Model file for the job. Use its own axes, mm. A direction names the side the tool comes from. Coordinates: 2 decimals unless noted, no trailing zeros. Order: outer loops, then holes, each group sorted by start corner. A loop starts at its lowest first (then second) coordinate and runs counter-clockwise, first axis right, second up. Notation, with made-up numbers: M 2.25,68 L 13.25,68 A12 cw 13.25,81 Z; hole C -8,51 d4. An arc over 180 degrees is marked long. Return JSON: item names as keys, results as strings.
Autodesk Inventor part; units mm, degrees
ref_plane "YZ Plane" through (0, 0, 0) normal (1, 0, 0) x (0, 1, 0)
ref_plane "XZ Plane" through (0, 0, 0) normal (0, 1, 0) x (-1, 0, 0)
ref_plane "XY Plane" through (0, 0, 0) normal (0, 0, 1) x (1, 0, 0)
sketch "Sketch1" plane through (0, 0, 0) normal (0, 1, 0) x (-1, 0, 0)
  circle A0 centre (0, 0) radius 11.5
  circle A1 centre (0, -22) radius 4.25
  line L0 (-21.5, 21.5) -> (21.5, 21.5)
  line L1 (21.5, 21.5) -> (21.5, -21.5)
  line L2 (21.5, -21.5) -> (-21.5, -21.5)
  line L3 (-21.5, -21.5) -> (-21.5, 21.5)
  line L4 (-21.5, 21.5) -> (21.5, -21.5) construction
  line L5 (21.5, 21.5) -> (-21.5, -21.5) construction
  line L6 (21.5, -21.5) -> (-21.5, -21.5)
  line L7 (-21.5, -21.5) -> (-21.5, -29.5)
  line L8 (-21.5, -29.5) -> (21.5, -29.5)
  line L9 (21.5, -29.5) -> (21.5, -21.5)
  circle A2 centre (15.5, 15.5) radius 1.8
  circle A3 centre (15.5, -15.5) radius 1.8
  circle A4 centre (-15.5, -15.5) radius 1.8
  circle A5 centre (-15.5, 15.5) radius 1.8
  point P0 (0, 0)
  dimension "d0" = 23
  dimension "d1" = 22
  dimension "d2" = 8.5
  dimension "d3" = 43
  dimension "d4" = 43
  dimension "d5" = 3.6
  dimension "d6" = 31
  dimension "d7" = 31
  dimension "d8" = 8
extrude "Extrusion1" add sketch "Sketch1" along normal blind 6 contours A1 L2 L9 L8 L7 | A1 L2 L3 L0 L1
sketch "Sketch2" plane through (0, 6, 0) normal (0, 1, 0) x (1, 0, 0)
  line L0 (-21.5, 29.5) -> (-21.5, -21.5)
  line L1 (-21.5, -21.5) -> (-26.5, -21.5)
  line L2 (-26.5, -21.5) -> (-26.5, 29.5)
  line L3 (-26.5, 29.5) -> (-21.5, 29.5)
  line L4 (-21.5, 29.5) -> (-21.5, -21.5)
  line L5 (21.5, -21.5) -> (26.5, -21.5)
  line L6 (26.5, -21.5) -> (26.5, 29.5)
  line L7 (26.5, 29.5) -> (21.5, 29.5)
  line L8 (21.5, 29.5) -> (21.5, -21.5)
  line L9 (-26.5, 29.5) -> (26.5, 29.5)
  line L10 (26.5, 29.5) -> (26.5, 24.5)
  line L11 (26.5, 24.5) -> (-26.5, 24.5)
  line L12 (-26.5, 24.5) -> (-26.5, 29.5)
  circle A0 centre (0, 22) radius 4.25
  line L13 (21.5, 29.5) -> (-21.5, 29.5)
  point P0 (0, 0)
  point P1 (-21.5, 24.5)
  point P2 (-3.4369, 24.5)
  point P3 (3.4369, 24.5)
  point P4 (21.5, 24.5)
  point P5 (21.5, 29.5)
  dimension "d11" = 5
  dimension "d12" = 5
  dimension "d13" = 5
extrude "Extrusion2" add sketch "Sketch2" against normal blind 43.081 contours L9 L8 L11 A0 L0 | L0 L11 L2 L3 | L0 L1 L2 L11 | L7 L6 L11 L8 | L11 L6 L5 L8
sketch "Sketch4" plane through (0, -37.081, 0) normal (0, -1, 0) x (1, 0, 0)
  line L0 (-26.5, 21.5) -> (26.5, 21.5)
  line L1 (26.5, 21.5) -> (41.5, 21.5)
  line L2 (41.5, 21.5) -> (41.5, -29.5)
  line L3 (41.5, -29.5) -> (26.5, -29.5)
  line L4 (26.5, -29.5) -> (26.5, 21.5)
  line L5 (-26.5, -29.5) -> (-26.5, 21.5)
  line L6 (-26.5, 21.5) -> (-41.5, 21.5)
  line L7 (-41.5, 21.5) -> (-41.5, -29.5)
  line L8 (-41.5, -29.5) -> (-26.5, -29.5)
  line L9 (-26.5, -29.5) -> (-26.5, 21.5)
  line L10 (-26.5, -29.5) -> (26.5, -29.5)
  circle A0 centre (-34, -5.25) radius 2.75
  circle A1 centre (34, -5.25) radius 2.75
  point P0 (0, 0)
  point P1 (-26.5, -29.5)
  dimension "d21" = 15
  dimension "d22" = 5.5
  dimension "d23" = 15
  dimension "d24" = 7.5
  dimension "d25" = 7.5
  dimension "d29" = 26.75
extrude "Extrusion3" add sketch "Sketch4" against normal blind 5 contours L5 L8 L7 L6 | L1 L2 L3 L4
sketch "Sketch5" plane through (0, -32.081, 0) normal (0, 1, 0) x (1, 0, 0)
  circle A0 centre (-34, 5.25) radius 2.75
  circle A1 centre (-34, 5.25) radius 5
  circle A2 centre (34, 5.25) radius 2.75
  circle A3 centre (34, 5.25) radius 5
  point P0 (0, 0)
  dimension "d30" = 10
extrude "Extrusion4" cut sketch "Sketch5" against normal blind 2 contours A1 | A2 | A3
sketch "Sketch7" plane through (26.5, 6, -29.5) normal (0, 0, -1) x (-1, 0, 0)
  line L0 (53, 0) -> (0, 0)
  line L1 (-15, -43.081) -> (-15, -38.081)
  line L2 (0, 0) -> (-15, -38.081)
  line L3 (-15, -38.081) -> (0, -38.081)
  line L4 (0, 0) -> (0, -38.081)
  line L5 (0, -38.081) -> (0, 0)
  line L6 (53, 0) -> (53, -38.081)
  line L7 (53, 0) -> (53, -38.081)
  line L8 (68, -38.081) -> (53, -38.081)
  line L9 (53, -38.081) -> (68, -38.081)
  line L10 (68, -38.081) -> (53, 0)
  point P0 (26.5, -6)
extrude "Extrusion5" add sketch "Sketch7" against normal blind 5
sketch "Sketch8" plane through (-21.5, 0, 21.5) normal (0, 0, 1) x (1, 0, 0)
  line L0 (-5, -32.081) -> (-20, -32.081)
  line L1 (-5, 6) -> (-5, -32.081)
  line L2 (-5, 6) -> (-20, -32.081)
  line L3 (63, -32.081) -> (48, -32.081)
  line L4 (63, -32.081) -> (48, 6)
  line L5 (48, -32.081) -> (48, 6)
  point P0 (21.5, 0)
extrude "Extrusion6" add sketch "Sketch8" against normal blind 5
fillet "Fillet1" radius 2 4 edges at (41.5, -32.081, -4) (-41.5, -32.081, -4) (-26.5, -32.081, -4) (26.5, -32.081, -4)
fillet "Fillet2" radius 2 8 edges at (-41.5, -34.581, 21.5) (-41.5, -34.581, -29.5) (41.5, -34.581, 21.5) (41.5, -34.581, -29.5) (34, -13.0405, 21.5) (34, -13.0405, -29.5) (-34, -13.0405, 21.5) (-34, -13.0405, -29.5)
sketch "Sketch10" plane through (0, -37.081, 0) normal (0, -1, 0) x (1, 0, 0)
  line L0 (-46.933, 35.2152) -> (46.933, 35.2152)
  line L1 (46.933, 35.2152) -> (46.933, -35.2152)
  line L2 (46.933, -35.2152) -> (-46.933, -35.2152)
  line L3 (-46.933, -35.2152) -> (-46.933, 35.2152)
  line L4 (-46.933, 35.2152) -> (46.933, -35.2152) construction
  line L5 (46.933, 35.2152) -> (-46.933, -35.2152) construction
  point P0 (0, 0)
sketch "Sketch9" plane through (0, 5, 0) normal (0, 1, 0) x (1, 0, 0)
  line L0 (41, 29) -> (41, -71)
  line L1 (41, 29) -> (-55.9789, 29)
  line L2 (-55.9789, 29) -> (-55.9789, -21)
  line L3 (-55.9789, -21) -> (41, -21)
  line L4 (41, -21) -> (41, 29)
  point P0 (0, 0)
  point P1 (41, -21)
properties part number "zmotorsupport"
Item 1: 3-axis set-ups, long thin cutter, end or side, ignore diameter. For faces 4 (the flat face through (-32, -18, -24.5)), 5 (the flat face through (36, -34.081, -3)), 6 (the cylindrical face through (40.9, -32.65, -4.29)): which of +Z, -Z, +X, -X, +Y, -Y reach the whole face in a straight line?
Check result:
{"face 4": "-X, +Y", "face 5": "+Y", "face 6": "+X, +Y"}
Item 2: Drop flat-ended pins along their axis: pin 1 Ø3 at (x, z) = (-34, -7.5) entering from +Y; pin 2 Ø6 at (x, z) = (-15.5, 15.5) entering from -Y; pin 3 Ø3.5 at (x, z) = (35, 5.5) entering from +Y; pin 4 Ø11 at (x, z) = (0, -22) entering from +Y. Give the stop position or say it passes through.
Check result:
{"pin 1": "stops at y = -34.08", "pin 2": "stops at y = 0", "pin 3": "stops at y = -32.08", "pin 4": "stops at y = 6"}
Item 3: Saw through at A-A (z = -22). Write the cut outline in (x, y), and give its area (3 significant figures).
Check result:
{"outline": "M -41.5,-37.08 L -21.5,-37.08 L -21.5,0 L -4.25,0 L -4.25,6 L -26.5,6 L -26.5,-30.08 A2 cw -28.5,-32.08 L -39.5,-32.08 A2 ccw -41.5,-34.08 Z; M 4.25,0 L 21.5,0 L 21.5,-37.08 L 41.5,-37.08 L 41.5,-34.08 A2 ccw 39.5,-32.08 L 28.5,-32.08 A2 cw 26.5,-30.08 L 26.5,6 L 4.25,6 Z", "area": "788 mm2"}
Item 4: Wall check: line 1 (Z direction, x = 15.5, y = 4.1); line 2 (X direction, y = -19, z = 1); line 3 (X direction, y = -33, z = -2). Give the ranges that are in metal, low to high.
Check result:
{"line 1": "z = -29.5 to -17.3, -13.7 to 13.7, 17.3 to 21.5", "line 2": "x = -26.5 to -21.5, 21.5 to 26.5", "line 3": "x = -41.18 to -37.8, -30.2 to -21.5, 21.5 to 30.2, 37.8 to 41.18"}
Item 5: Saw through at B-B (x = 15.5). Write the cut outline in (y, z).
Check result:
{"outline": "M -37.08,-29.5 L 6,-29.5 L 6,-17.3 L 0,-17.3 L 0,-24.5 L -37.08,-24.5 Z; M 0,-13.7 L 6,-13.7 L 6,13.7 L 0,13.7 Z; M 0,17.3 L 6,17.3 L 6,21.5 L 0,21.5 Z"}
Item 6: Saw through at D-D (x = 6). Write the cut outline in (y, z), and give its area (3 significant figures).
Check result:
{"outline": "M -37.08,-29.5 L 6,-29.5 L 6,-9.81 L 0,-9.81 L 0,-24.5 L -37.08,-24.5 Z; M 0,9.81 L 6,9.81 L 6,21.5 L 0,21.5 Z", "area": "374 mm2"}
Item 7: Saw through at C-C (z = -15.5). Write the cut outline in (x, y).
Check result:
{"outline": "M -41.5,-37.08 L -21.5,-37.08 L -21.5,0 L -17.3,0 L -17.3,6 L -26.5,6 L -26.5,-30.08 A2 cw -28.5,-32.08 L -39.5,-32.08 A2 ccw -41.5,-34.08 Z; M -13.7,0 L 13.7,0 L 13.7,6 L -13.7,6 Z; M 17.3,0 L 21.5,0 L 21.5,-37.08 L 41.5,-37.08 L 41.5,-34.08 A2 ccw 39.5,-32.08 L 28.5,-32.08 A2 cw 26.5,-30.08 L 26.5,6 L 17.3,6 Z"}
Item 8: Pull direction X, two halves, no side cores. Call faces 1 (the cylindrical face through (33.403, -13.166, -28.93)), 2 (the flat face through (21.5, -18, -2)), 3 (the flat face through (-26.5, -12, -4)): +X half, -X half, draft (parallel to the pull), parting line (faces both ways), or undercut.
Check result:
{"face 1": "+X half", "face 2": "undercut", "face 3": "-X half"}
